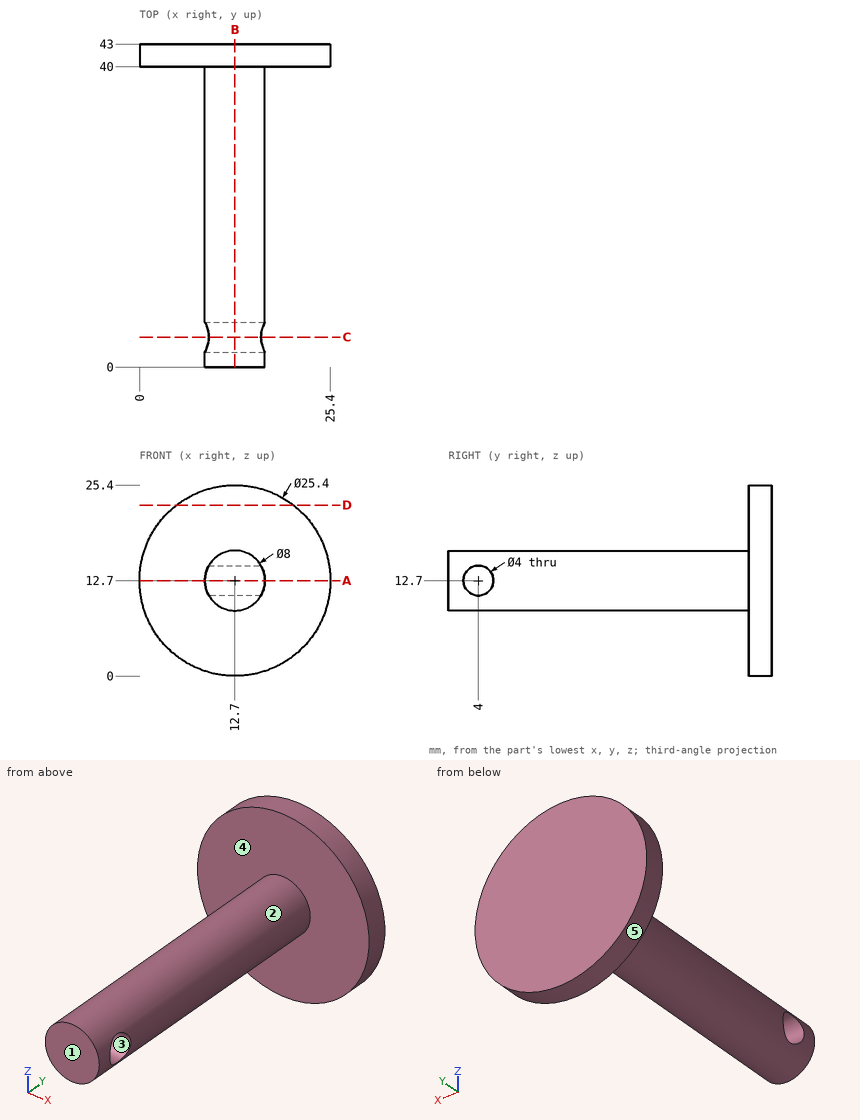
Here's the drawing with two shaded views (mm, measured from the low corner). I have some questions. A direction names the side the tool comes from. Give positions to 0.01 mm unless a question says otherwise; leave off trailing zeros. Order: outer loops, then holes, each group sorted by start corner. A loop starts at its lowest first (then second) coordinate and runs counter-clockwise, first axis right, second up. Notation, with made-up numbers: M -32.5,36.5 L 15.5,36.5 A33 ccw 15.5,73.5 Z; hole C 71.5,69 d8. An arc over 180 degrees is marked long. One line per item, written item: value.
1) Please list where these lines run through material, in increasing order: line 1 along Y through (x, z) = (14.5, 12.7); line 2 along Y through (x, z) = (12, 22); line 3 along X through (y, z) = (11.5, 14.75).
Answer sheet:
line 1: y = 0 to 2, 6 to 43
line 2: y = 40 to 43
line 3: x = 9.27 to 16.13
2) I want a section at D-D, the plane z = 22.75. List the corners of the cut face in (x, y) for me, plus the area to 3 significant figures.
Answer sheet:
outline: M 4.94,40 L 20.46,40 L 20.46,43 L 4.94,43 Z
area: 46.6 mm^2
3) I want a section at A-A, the plane z = 12.7. List the corners of the cut face in (x, y) for me.
Answer sheet:
outline: M 0,40 L 8.7,40 L 8.7,6 L 16.7,6 L 16.7,40 L 25.4,40 L 25.4,43 L 0,43 Z; M 8.7,0 L 16.7,0 L 16.7,2 L 8.7,2 Z
4) I want a section at C-C, the plane y = 4. List the corners of the cut face in (x, z) for me.
Answer sheet:
outline: M 9.24,10.7 A4 ccw 16.16,10.7 Z; M 9.24,14.7 L 16.16,14.7 A4 ccw Z
5) On a 3-axis mill with a long thin cutter (end or side, diameter ignored), from which of +Z, -Z, +X, -X, +Y, -Y can I reach the whole of each face in a straight line? I mean the marked faces 1 and 2. Say none if no direction works.
Answer sheet:
face 1: +Z, -Z, +X, -X, -Y
face 2: -Y
6) For P1, Ø1.5, axis at x = 7, y = 37, coming from the +Z side; P2, Ø12, axis at y = 9.5, z = 9.5, coming from the +X side; P3, Ø5, axis at x = 10, y = 18, coming from the -Z side (3 decimals); P4, Ø1.5, axis at x = 7, z = 6, coming from the -Y side, each with a flat end and sliding along its axis, tell me the tip position at first contact or that it passes through.
Answer sheet:
P1: passes through
P2: stops at x = 16.7
P3: stops at z = 8.705
P4: stops at y = 40
7) I want a section at B-B, the plane x = 12.7. List the corners of the cut face in (y, z) for me, plus the area to 3 significant figures.
Answer sheet:
outline: M 0,8.7 L 40,8.7 L 40,0 L 43,0 L 43,25.4 L 40,25.4 L 40,16.7 L 0,16.7 Z; hole C 4,12.7 d4
area: 384 mm^2
8) We'd pull the mould along Z, two halves only. Please class the marked faces 3, 4 and 5: released by +Z, released by -Z, zero draft, split by the parting line, or undercut.
Answer sheet:
face 3: undercut
face 4: zero draft
face 5: split by the parting line
